from build123d import *

# Parameters (mm, degrees)
SKETCH1_W               = 1219.2
SKETCH1_H               = 2102.64375
BOSS_EXTRUDE1_DEPTH     = 5.55625
CUT_EXTRUDE1_DEPTH      = 1216.286269472
CUT_EXTRUDE1_DEPTH_BACK = 1216.286269472
SKETCH2_W               = 508
SKETCH2_H               = 508


with BuildPart() as part:
    # Sketch1 → Boss-Extrude1 (new body)
    with BuildSketch(Plane(origin=(0, 0, 0), x_dir=(1, 0, 0), z_dir=(0, 1, 0))):
        Rectangle(SKETCH1_W, SKETCH1_H)
    extrude(amount=BOSS_EXTRUDE1_DEPTH)

    # Sketch2 → Cut-Extrude1 (cut, two sides: drawn at the far end of the back side and taken through both)
    with BuildSketch(Plane(origin=(0, 0, 0), x_dir=(-1, 0, 0), z_dir=(0, -1, 0)).offset(-CUT_EXTRUDE1_DEPTH_BACK)):
        with Locations((0, 492.521875)):
            Rectangle(SKETCH2_W, SKETCH2_H)
        with Locations((0, -155.178125)):
            Rectangle(SKETCH2_W, SKETCH2_H)
    extrude(amount=CUT_EXTRUDE1_DEPTH + CUT_EXTRUDE1_DEPTH_BACK, mode=Mode.SUBTRACT)


solid = part.part
Work out the finished part from the listing and answer in its coordinate system (mm). Round coordinates to 2 decimals unless told otherwise and drop trailing zeros. Loops run counter-clockwise (first coordinate to the right, second up) from the corner with the lowest first, then second, coordinate; pieces in that order, holes last. Notation, with made-up numbers: (78, 21) -> (108, 21) arc R19 cw to (108, 56) -> close; hole circle Ø7 at (44.25, -2). An arc over 180 degrees is marked (long way). Use one line per item in the form item = value.
(1) Find section B-B on z = -445.5. Give the vertices of the cut face in (x, y).
Answer list:
outline = (-609.6, 0) -> (-254, 0) -> (-254, 5.56) -> (-609.6, 5.56) -> close; (254, 0) -> (609.6, 0) -> (609.6, 5.56) -> (254, 5.56) -> close
(2) Find section A-A on x = 179. Give the vertices of the cut face in (y, z), then the cut area to 3 significant figures.
Answer list:
outline = (0, -1051.32) -> (5.56, -1051.32) -> (5.56, -746.52) -> (0, -746.52) -> close; (0, -238.52) -> (5.56, -238.52) -> (5.56, -98.82) -> (0, -98.82) -> close; (0, 409.18) -> (5.56, 409.18) -> (5.56, 1051.32) -> (0, 1051.32) -> close
area = 6,040 mm2
(3) Find section C-C on y = 1.2. Give the vertices of the cut face in (x, z), then the cut area to 3 significant figures.
Answer list:
outline = (-609.6, -1051.32) -> (609.6, -1051.32) -> (609.6, 1051.32) -> (-609.6, 1051.32) -> close; hole (-254, -746.52) -> (254, -746.52) -> (254, -238.52) -> (-254, -238.52) -> close; hole (-254, -98.82) -> (254, -98.82) -> (254, 409.18) -> (-254, 409.18) -> close
area = 2,050,000 mm2
(4) Straight lines are drawn through the part: line 1 (Z direction, x = -200.5, y = 2.95); line 2 (X direction, y = 1.65, z = -332). For each, find the intervals that lie inside material, in ascending order.
Answer list:
line_1 = -1051.32 to -746.52, -238.52 to -98.82, 409.18 to 1051.32
line_2 = -609.6 to -254, 254 to 609.6
(5) For a pull along Y with two mould halves and no side action, classify faces 1 (the flat face through (262, 0, -15)), 2 (the flat face through (262, 5.556, -15)) as released by +Y, released by -Y, zero draft, split by the parting line, or undercut.
Answer list:
face_1 = released by -Y
face_2 = released by +Y
